Read the model definition and answer for the solid it produces. Units are mm, in the model's axes. A direction names the side the tool comes from. Round coordinates to 2 decimals unless told otherwise and drop trailing zeros. Order: outer loops, then holes, each group sorted by start corner. A loop starts at its lowest first (then second) coordinate and runs counter-clockwise, first axis right, second up. Notation, with made-up numbers: (42.25, 47) - (99.25, 47) arc R22 cw to (99.25, 67) - close; hole circle Ø4 at (8, -18.5). An arc over 180 degrees is marked (long way). Answer as a JSON object with one key per item and string values. Group by question number.
Q1. Given pin 1 Ø8 at (x, y) = (32.5, 13.5) entering from +Z; pin 2 Ø8 at (x, y) = (-26.5, 13) entering from +Z; pin 3 Ø10 at (x, y) = (98, 15.5) entering from -Z; pin 4 Ø2 at (x, z) = (59.5, 41) entering from -Y, each flat-ended and moving along its own axis, determine where each tip first touches the part or whether it passes through.
Q2. A cutting plane is placed at C-C on y = 10. Determine the outline of the cut face in (x, z).
Q3. Consider line 1 (X direction, y = 8.5, z = 0); line 2 (Z direction, x = 0, y = 1.6) (3 decimals); line 3 (Z direction, x = 0, y = 10.5). Determine where each line is inside the solid, lowest interval first.
Q4. A cutting plane is placed at A-A on z = 0. Determine the outline of the cut face in (x, y) (3 decimals).
Q5. A cutting plane is placed at D-D on z = 43. Determine the outline of the cut face in (x, y) (3 decimals), and give its area (3 significant figures).
Q6. A cutting plane is placed at B-B on x = 0. Determine the outline of the cut face in (y, z) (3 decimals).
Q7. The mould has two halves that part along X. Classify faces 1 (the flat face through (56, 11.001, 36.797)), 2 (the cylindrical face through (120.772, 11.001, -0.517)), 3 (the cylindrical face through (-53.957, 1.565, 1.398)), 4 (the flat face through (16, 3.175, 1)): pulls with the +X half, pulls with the -X half, needs draft (parallel to the pull), parting line crosses it, or undercut.
Q8. A tool of negligible diameter and unlimited length cuts with its end or side. For faces 5 (the flat face through (33, 19.05, -44)), 6 (the cylindrical face through (117.598, 11.001, -0.459)), from which of +Z, -Z, +X, -X, +Y, -Y can it reach the whole face along a straight path? Write none if from no direction.
Autodesk Inventor part; units mm, degrees
ref_plane "YZ Plane" through (0, 0, 0) normal (1, 0, 0) x (0, 1, 0)
ref_plane "XZ Plane" through (0, 0, 0) normal (0, 1, 0) x (-1, 0, 0)
ref_plane "XY Plane" through (0, 0, 0) normal (0, 0, 1) x (1, 0, 0)
sketch "Sketch1" plane through (0, 0, 0) normal (0, 1, 0) x (-1, 0, 0)
  circle A0 centre (0, 0) radius 53.975
  circle A1 centre (-92.202, 0) radius 28.575
  line L0 (-14.8691, 51.8865) -> (-100.0739, 27.4693)
  line L1 (-100.0739, -27.4693) -> (-14.8691, -51.8865)
  dimension "d0" = 107.95
  dimension "d1" = 57.15
  dimension "d2" = 92.202
  dimension "d3" = 0
extrude "Extrusion1" add sketch "Sketch1" along normal blind 3.175
sketch "Sketch3" plane through (0, 3.175, 0) normal (0, 1, 0) x (1, 0, 0)
  point P0 (0, 0)
  point P1 (0, 0)
sketch "Sketch4" plane through (0, 3.175, 0) normal (0, 1, 0) x (1, 0, 0)
  arc A0 (100.0739, -27.4693) -> (100.0739, 27.4693) centre (92.202, 0) ccw
  point P0 (0, 0)
hole "Hole1" at (0, 3.175, 0) direction (0, -1, 0) diameter 13.208 end through all
hole "Hole2" at (92.202, 3.175, 0) direction (0, -1, 0) diameter 7.112 end through all
sketch "Sketch5" plane through (0, 3.175, 0) normal (0, 1, 0) x (1, 0, 0)
  circle A0 centre (0, 0) radius 50.8
  circle A1 centre (92.202, 0) radius 3.556
  circle A2 centre (92.202, 0) radius 25.4
  line L0 (13.9945, -48.8344) -> (99.1992, -24.4172)
  line L1 (13.9945, 48.8344) -> (99.1992, 24.4172)
  line L2 (14.8691, -51.8865) -> (100.0739, -27.4693)
  arc A3 (14.8691, 51.8865) -> (14.8691, -51.8865) centre (0, 0) ccw
  line L3 (100.0739, 27.4693) -> (14.8691, 51.8865)
  arc A4 (100.0739, -27.4693) -> (100.0739, 27.4693) centre (92.202, 0) ccw
  dimension "d20" = 101.6
  dimension "d21" = 50.8
extrude "Extrusion2" add sketch "Sketch5" along normal blind 15.875 contours A3 L3 A4 L2
properties part number "chain guard"
Result set:
{
 "1": {"pin 1": "stops at z = 47.98", "pin 2": "stops at z = 49.06", "pin 3": "stops at z = -29.5", "pin 4": "passes through"},
 "2": {"outline": "(14.87, -51.89) - (100.07, -27.47) arc R28.57 ccw to (100.07, 27.47) - (14.87, 51.89) arc R53.97 ccw (long way) to start; hole (13.99, -48.83) - (99.2, -24.42) arc R25.4 ccw to (99.2, 24.42) - (13.99, 48.83) arc R50.8 ccw (long way) to start"},
 "3": {"line 1": "x = -53.97 to -50.8, 117.6 to 120.78", "line 2": "z = -53.975 to -6.604, 6.604 to 53.975", "line 3": "z = -53.97 to -50.8, 50.8 to 53.97"},
 "4": {"outline": "(-53.975, 0) - (-6.604, 0) - (-6.604, 3.175) - (-50.8, 3.175) - (-50.8, 19.05) - (-53.975, 19.05) - close; (6.604, 0) - (88.646, 0) - (88.646, 3.175) - (6.604, 3.175) - close; (95.758, 0) - (120.777, 0) - (120.777, 19.05) - (117.602, 19.05) - (117.602, 3.175) - (95.758, 3.175) - close"},
 "5": {"outline": "(-32.624, 0) - (45.879, 0) - (45.879, 19.05) - (34.354, 19.05) - (34.354, 3.175) - (-27.049, 3.175) - (-27.049, 19.05) - (-32.624, 19.05) - close", "area": "521 mm²"},
 "6": {"outline": "(0, -53.975) - (19.05, -53.975) - (19.05, -50.8) - (3.175, -50.8) - (3.175, -6.604) - (0, -6.604) - close; (0, 6.604) - (3.175, 6.604) - (3.175, 50.8) - (19.05, 50.8) - (19.05, 53.975) - (0, 53.975) - close"},
 "7": {"face 1": "undercut", "face 2": "pulls with the +X half", "face 3": "parting line crosses it", "face 4": "undercut"},
 "8": {"face 5": "+Z, -Z, +X, -X, +Y", "face 6": "+Y"}
}
